Geometry check sheet. Reference: the model listing, model coordinates, mm. Face numbers are marked on the shaded views. A direction names the side the tool comes from. Coordinates: 2 decimals unless noted, no trailing zeros. Write each loop counter-clockwise with the first axis right and the second up, starting at its lowest first coordinate (ties: lowest second). Pieces come first, ordered by that corner, then holes. Notation, with made-up numbers: M 34.5,6.25 L 81.5,6.25 A35 cw 81.5,43.25 Z; hole C 2.5,39 d1. An arc over 180 degrees is marked long. Write item = value, one per line. Start each with the question number.
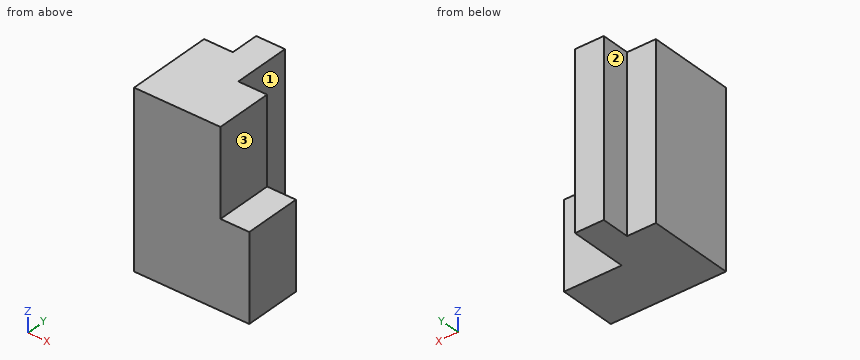
```python
from build123d import *

# Parameters (mm, degrees)
SKETCH1_W           = 40
SKETCH1_H           = 40
BOSS_EXTRUDE1_DEPTH = 60
SKETCH2_W           = 20
SKETCH2_H           = 60
CUT_EXTRUDE1_DEPTH  = 20
SKETCH3_W           = 10
SKETCH3_H           = 30
CUT_EXTRUDE2_DEPTH  = 20
SKETCH4_W           = 10
SKETCH4_H           = 60
CUT_EXTRUDE3_DEPTH  = 10


with BuildPart() as part:
    # Sketch1 → Boss-Extrude1 (new body)
    with BuildSketch(Plane.XY):
        with Locations((20, 20)):
            Rectangle(SKETCH1_W, SKETCH1_H)
    extrude(amount=BOSS_EXTRUDE1_DEPTH)

    # Sketch2 → Cut-Extrude1 (cut)
    with BuildSketch(Plane(origin=(0, 40, 0), x_dir=(1, 0, 0), z_dir=(0, 1, 0))):
        with Locations((30, -30)):
            Rectangle(SKETCH2_W, SKETCH2_H)
    extrude(amount=-CUT_EXTRUDE1_DEPTH, mode=Mode.SUBTRACT)

    # Sketch3 → Cut-Extrude2 (cut)
    with BuildSketch(Plane(origin=(0, 20, 0), x_dir=(1, 0, 0), z_dir=(0, 1, 0))):
        with Locations((35, -45)):
            Rectangle(SKETCH3_W, SKETCH3_H)
    extrude(amount=-CUT_EXTRUDE2_DEPTH, mode=Mode.SUBTRACT)

    # Sketch4 → Cut-Extrude3 (cut)
    with BuildSketch(Plane(origin=(0, 40, 0), x_dir=(1, 0, 0), z_dir=(0, 1, 0))):
        with Locations((5, -30)):
            Rectangle(SKETCH4_W, SKETCH4_H)
    extrude(amount=-CUT_EXTRUDE3_DEPTH, mode=Mode.SUBTRACT)


solid = part.part
```
Q1. Cross-section at C-C on x = 5.5. Enter the section's corners in (y, z), and give its area (3 significant figures).
Q2. Set-up check for the marked faces 1, 2 and 3: record each of +Z, -Z, +X, -X, +Y, -Y from which the full face is reachable in a straight line by a thin tool's end or side.
Q3. Cross-section at D-D on z = 39. Enter the section's corners in (x, y), and give its area (3 significant figures).
Q4. Scan lines: L1, parallel to X at y = 32, z = 6.5; L2, parallel to X at y = 23, z = 50.5; L3, parallel to Y at x = 6.5, z = 17.5. Record each from-to range of solid material in increasing order.
Q5. Gauge pin test, flat ends, axial feed: pin 1 (8 mm diameter, centred on x = 37, y = 7.5, fed in from +Z); pin 2 (22 mm diameter, centred on y = 31.5, z = 23.5, fed in from +X); pin 3 (16 mm diameter, centred on x = 29.5, z = 29, fed in from +Y). Record the tip position at first contact, or that the pin passes through.
Q6. Cross-section at A-A on z = 12. Enter the section's corners in (x, y), and give its area (3 significant figures).
Q7. Cross-section at B-B on y = 25.5. Enter the section's corners in (x, z), and give its area (3 significant figures).
Values found:
q1.outline = M 0,0 L 30,0 L 30,60 L 0,60 Z
q1.area = 1,800 mm²
q2.face_1 = +Z, -Z, +X, +Y
q2.face_2 = +Z, -Z, -X, +Y
q2.face_3 = +Z, +X, +Y, -Y
q3.outline = M 0,0 L 30,0 L 30,20 L 20,20 L 20,40 L 10,40 L 10,30 L 0,30 Z
q3.area = 900 mm²
q4.L1 = 10 to 20
q4.L2 = 0 to 20
q4.L3 = 0 to 30
q5.pin_1 = 30
q5.pin_2 = 20
q5.pin_3 = 20
q6.outline = M 0,0 L 40,0 L 40,20 L 20,20 L 20,40 L 10,40 L 10,30 L 0,30 Z
q6.area = 1,100 mm²
q7.outline = M 0,0 L 20,0 L 20,60 L 0,60 Z
q7.area = 1,200 mm²
